Build history of the part. All positions in model axes, mm. Coordinates: 2 decimals unless noted, no trailing zeros. Write each loop counter-clockwise with the first axis right and the second up, starting at its lowest first coordinate (ties: lowest second). Pieces come first, ordered by that corner, then holes. Notation, with made-up numbers: M 50,-11.75 L 59,-11.75 A9 cw 59,-3.75 Z; hole C 37,62 d7. An arc over 180 degrees is marked long. Use CSV: the item, a comma, the result in double quotes. Start each with the question number.
```python
from build123d import *

# Parameters (mm, degrees)
SKETCH_2_R          = 0.29
SKETCH_2_R_2        = 0.15
EXTRUDE_1_DEPTH     = 0.2
EXTRUDE_3_DEPTH     = 0.2
CUT_EXTRUDE_START   = -0.2
CUT_EXTRUDE_2_DEPTH = 0.2


# Read off the part's stored shape, not the designer's step: 切除-拉伸2
with BuildPart() as part:
    # 草图2 → 凸台-拉伸1 (new body)
    with BuildSketch(Plane.XY):
        Circle(SKETCH_2_R)
        Circle(SKETCH_2_R_2, mode=Mode.SUBTRACT)
    extrude(amount=EXTRUDE_1_DEPTH)

    # 草图3 → 凸台-拉伸3 (add)
    with BuildSketch(Plane.XY.offset(0.2)):
        Polygon((0, 0), (0, 9.030931314), (-0.203353638, 6.330931314), (-0.091221417, 6.330931314), (-0.091221417, 0), align=None)
    extrude_3 = extrude(amount=-EXTRUDE_3_DEPTH)

    # 镜向1: 凸台-拉伸3 across plane
    add(extrude_3.mirror(Plane(origin=(0, 0, 0), x_dir=(0, 0, 1), z_dir=(1, 0, 0))))

    # 切除-拉伸2 outline → 切除-拉伸2 (cut)
    with BuildSketch(Plane.XY.offset(0.2).offset(CUT_EXTRUDE_START)):
        with BuildLine():
            Line((0.091221417, 0), (0.091221417, 0.11907415))
            ThreePointArc((0.091221417, 0.11907415), (0, 0.15), (-0.091221417, 0.11907415))
            Line((-0.091221417, 0.11907415), (-0.091221417, 0))
            Line((-0.091221417, 0), (0.091221417, 0))
        make_face()
    extrude(amount=CUT_EXTRUDE_2_DEPTH, mode=Mode.SUBTRACT)


solid = part.part
```
1. Drill centre line: line 1 along X through (y, z) = (4.5, 0.15). Where is it in solid material? Low to high. Write a range as from..to.
2. Slice it at D-D (y = 7). List the corners of the cut face in (x, z), and give its area (3 significant figures).
3. Slice it at C-C (y = 4). List the corners of the cut face in (x, z), and give its area (3 significant figures).
4. Slice it at A-A (y = 0). List the corners of the cut face in (x, z), and give its area (3 significant figures).
5. Slice it at B-B (z = 0.1). List the corners of the cut face in (x, y).
Established:
1,line 1,"x = -0.09..0.09"
2,outline,"M -0.15,0 L 0.15,0 L 0.15,0.2 L -0.15,0.2 Z"
2,area,"0.0612 mm2"
3,outline,"M -0.09,0 L 0.09,0 L 0.09,0.2 L -0.09,0.2 Z"
3,area,"0.0365 mm2"
4,outline,"M -0.29,0 L -0.15,0 L -0.15,0.2 L -0.29,0.2 Z; M 0.15,0 L 0.29,0 L 0.29,0.2 L 0.15,0.2 Z"
4,area,"0.0560 mm2"
5,outline,"M -0.2,6.33 L -0.09,6.33 L -0.09,0.28 A0.29 ccw long 0.09,0.28 L 0.09,6.33 L 0.2,6.33 L 0,9.03 Z; hole C 0,0 d0.3"
